from build123d import *

# Parameters (mm, degrees)
EXTRUDE_1_DEPTH     = 7
SKETCH_2_W          = 7
SKETCH_2_H          = 24
EXTRUDE_2_DEPTH     = 10
FILLET_1_R          = 10
FILLET_2_R          = 10
SKETCH_3_R          = 2.5
CUT_EXTRUDE_1_DEPTH = 104.07764064
FILLET_3_R          = 10
FILLET_4_R          = 10
FILLET_5_R          = 10
FILLET_6_R          = 10
FILLET_8_R          = 5
FILLET_9_R          = 5
SKETCH_4_R          = 2.5
CUT_EXTRUDE_2_DEPTH = 104.077640708
SKETCH_5_R          = 2.5
CUT_EXTRUDE_3_DEPTH = 104.990384238
FILLET_10_R         = 5
FILLET_11_R         = 5


with BuildPart() as part:
    # 草图1 → 凸台-拉伸1 (new body)
    with BuildSketch(Plane(origin=(0, 0, 0), x_dir=(1, 0, 0), z_dir=(0, 1, 0))):
        Polygon((0, 0), (7, 0), (7, -43), (35, -43), (63, -43), (63, 0), (70, 0), (70, -75), (0, -75), align=None)
    extrude(amount=EXTRUDE_1_DEPTH)

    # 草图2 → 凸台-拉伸2 (add)
    with BuildSketch(Plane.XZ):
        with Locations((3.5, 12)):
            Rectangle(SKETCH_2_W, SKETCH_2_H)
        with Locations((66.5, 12)):
            Rectangle(SKETCH_2_W, SKETCH_2_H)
    extrude(amount=EXTRUDE_2_DEPTH)

    # 圆角1
    fillet_1_edges = [part.edges().sort_by_distance(p)[0] for p in [
        (3.5, 0, 24),
    ]]
    fillet(fillet_1_edges, radius=FILLET_1_R - 0.0001)  # a hair under: the kernel refuses the full size

    # 圆角2
    fillet_2_edges = [part.edges().sort_by_distance(p)[0] for p in [
        (66.5, 0, 24),
    ]]
    fillet(fillet_2_edges, radius=FILLET_2_R - 0.0001)  # a hair under: the kernel refuses the full size

    # 草图3 → 切除-拉伸1 (cut, through all)
    with BuildSketch(Plane(origin=(70, 0, 0), x_dir=(0, 0, -1), z_dir=(1, 0, 0))):
        with Locations((-12, -4)):
            Circle(SKETCH_3_R)
    extrude(amount=-CUT_EXTRUDE_1_DEPTH, mode=Mode.SUBTRACT)

    # 圆角3
    fillet_3_edges = [part.edges().sort_by_distance(p)[0] for p in [
        (3.5, 7, 0),
    ]]
    fillet(fillet_3_edges, radius=FILLET_3_R)

    # 圆角4
    fillet_4_edges = [part.edges().sort_by_distance(p)[0] for p in [
        (66.5, 7, 0),
    ]]
    fillet(fillet_4_edges, radius=FILLET_4_R)

    # 圆角5
    fillet_5_edges = [part.edges().sort_by_distance(p)[0] for p in [
        (7, 3.5, 43),
    ]]
    fillet(fillet_5_edges, radius=FILLET_5_R)

    # 圆角6
    fillet_6_edges = [part.edges().sort_by_distance(p)[0] for p in [
        (63, 3.5, 43),
    ]]
    fillet(fillet_6_edges, radius=FILLET_6_R)

    # 圆角8
    fillet_8_edges = [part.edges().sort_by_distance(p)[0] for p in [
        (66.5, -10, 0),
    ]]
    fillet(fillet_8_edges, radius=FILLET_8_R)

    # 圆角9
    fillet_9_edges = [part.edges().sort_by_distance(p)[0] for p in [
        (3.5, -10, 0),
    ]]
    fillet(fillet_9_edges, radius=FILLET_9_R)

    # 草图4 → 切除-拉伸2 (cut, through all)
    with BuildSketch(Plane(origin=(70, 0, 0), x_dir=(0, 0, -1), z_dir=(1, 0, 0))):
        with Locations((-4, -4)):
            Circle(SKETCH_4_R)
        with Locations((-20, -4)):
            Circle(SKETCH_4_R)
    extrude(amount=-CUT_EXTRUDE_2_DEPTH, mode=Mode.SUBTRACT)

    # 草图5 → 切除-拉伸3 (cut, through all)
    with BuildSketch(Plane(origin=(0, 7, 0), x_dir=(1, 0, 0), z_dir=(0, 1, 0))):
        with Locations(Location((19.2, -70, 0), (0, 0, 270))):
            Circle(SKETCH_5_R)
        with Locations(Location((50.8, -70, 0), (0, 0, 270))):
            Circle(SKETCH_5_R)
    extrude(amount=-CUT_EXTRUDE_3_DEPTH, mode=Mode.SUBTRACT)

    # 圆角10
    fillet_10_edges = [part.edges().sort_by_distance(p)[0] for p in [
        (0, 3.5, 75),
    ]]
    fillet(fillet_10_edges, radius=FILLET_10_R)

    # 圆角11
    fillet_11_edges = [part.edges().sort_by_distance(p)[0] for p in [
        (70, 3.5, 75),
    ]]
    fillet(fillet_11_edges, radius=FILLET_11_R)


solid = part.part
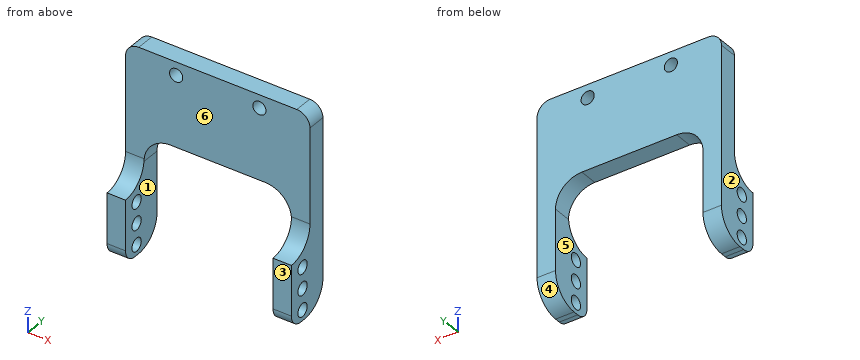
Input: part model. Units: mm. Frame: model coordinates. Face numbers are marked on the shaded views. A direction names the side the tool comes from. Give positions to 0.01 mm unless a question says otherwise; leave off trailing zeros. Write each loop counter-clockwise with the first axis right and the second up, starting at its lowest first coordinate (ties: lowest second). Pieces come first, ordered by that corner, then holes. Notation, with made-up numbers: (-32.75, 79.25) -> (-25.75, 79.25) arc R24 cw to (-25.75, 118.25) -> close; hole circle Ø1 at (28.5, 50). An arc over 180 degrees is marked (long way). Use one line per item in the form item = value. Start each with the question number.
1) Draft query along X for the marked faces 1, 2 and 3. Return one class per face: pulls with the +X half, pulls with the -X half, needs draft (parallel to the pull), parting line crosses it, or undercut.
2) Pin query (flat end, axial travel): pin 1 (5 mm diameter, centred on x = 14.5, z = 62.5, fed in from -Y); pin 2 (2 mm diameter, centred on x = 38.5, y = 5, fed in from -Z). Return the tip coordinate at first contact, or that it passes through.
3) Section query A-A on z = 20. Return the cut outline in (x, y).
4) Section query D-D on x = 35. Return the cut outline in (y, z).
5) Section query B-B on y = -8.5. Return the cut outline in (x, z), then the cut area to 3 significant figures.
6) Set-up query: the marked faces 4, 5 and 6. Return all of +Z, -Z, +X, -X, +Y, -Y with unobstructed straight access to the full face (end or side cutting, diameter ignored); none if empty.
7) Ray query, probe 1 along X at (y, z) = (3.75, 70); probe 2 along Y at (x, z) = (65.5, 20); probe 3 along X at (y, z) = (4, 3). Return the intervals inside material, ascending. Write a range as from..to.
8) Section query C-C on y = 5.5. Return the cut outline in (x, z), then the cut area to 3 significant figures.
Outcome:
q1.face_1 = undercut
q1.face_2 = pulls with the -X half
q1.face_3 = needs draft
q2.pin_1 = 0
q2.pin_2 = 43
q3.outline = (0, -10) -> (7, -10) -> (7, -6.5) -> (0, -6.5) -> close; (0, -1.5) -> (7, -1.5) -> (7, 7) -> (0, 7) -> close; (63, -10) -> (70, -10) -> (70, -6.5) -> (63, -6.5) -> close; (63, -1.5) -> (70, -1.5) -> (70, 7) -> (63, 7) -> close
q4.outline = (0, 43) -> (7, 43) -> (7, 75) -> (0, 75) -> close
q5.outline = (0, 1.43) -> (7, 1.43) -> (7, 24.11) -> (0, 24.11) -> close; (63, 1.43) -> (70, 1.43) -> (70, 24.11) -> (63, 24.11) -> close
q5.area = 318 mm^2
q6.face_4 = -Z, +X, -X, +Y
q6.face_5 = -Z, +Y, -Y
q6.face_6 = +Z, +X, -X, -Y
q7.probe_1 = 0..16.7, 21.7..48.3, 53.3..70
q7.probe_2 = -10..-6.5, -1.5..7
q7.probe_3 = 0..7, 63..70
q8.outline = (0, 4.73) -> (7, 4.73) -> (7, 33) arc R10 cw to (17, 43) -> (53, 43) arc R10 cw to (63, 33) -> (63, 4.73) -> (70, 4.73) -> (70, 70) arc R5 ccw to (65, 75) -> (5, 75) arc R5 ccw to (0, 70) -> close; hole circle Ø5 at (19.2, 70); hole circle Ø5 at (50.8, 70)
q8.area = 2,770 mm^2
